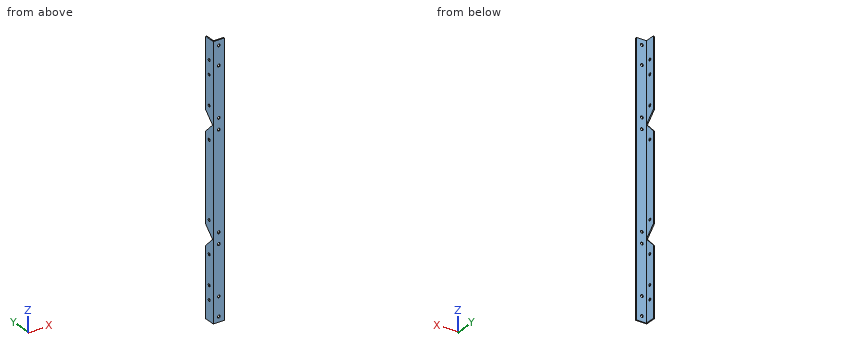
```python
from build123d import *

# Parameters (mm, degrees)
BOSS_EXTRUDE1_DEPTH = 208.28
SKETCH2_R           = 2.38125
CUT_EXTRUDE1_DEPTH  = 1.778
SKETCH3_W           = 1.778
SKETCH3_H           = 17.272
BOSS_EXTRUDE2_DEPTH = 20.32
SKETCH4_R           = 2.38125
CUT_EXTRUDE2_DEPTH  = 1.778


with BuildPart() as part:
    # Sketch1 → Boss-Extrude1 (new body)
    with BuildSketch(Plane.XY):
        Polygon((0, 0), (0, 17.272), (-1.778, 17.272), (-1.778, -1.778), (17.272, -1.778), (17.272, 0), align=None)
    boss_extrude1 = extrude(amount=BOSS_EXTRUDE1_DEPTH)

    # Sketch2 → Cut-Extrude1 (cut)
    with BuildSketch(Plane(origin=(0, 0, 0), x_dir=(0, 0, -1), z_dir=(1, 0, 0))):
        with Locations(Location((-194.31, 8.636, 0), (0, 0, 90))):
            Circle(SKETCH2_R)
        with Locations(Location((-170.434, 8.636, 0), (0, 0, 90))):
            Circle(SKETCH2_R)
        with Locations(Location((-120.269, 8.636, 0), (0, 0, 90))):
            Circle(SKETCH2_R)
        with Locations(Location((-64.897, 8.636, 0), (0, 0, 90))):
            Circle(SKETCH2_R)
        Polygon((-92.583, 0), (-109.855, 17.272), (-75.311, 17.272), align=None)
    cut_extrude1 = extrude(amount=-CUT_EXTRUDE1_DEPTH, mode=Mode.SUBTRACT)

    # Sketch3 → Boss-Extrude2 (add)
    with BuildSketch(Plane.XY.offset(208.28)):
        Polygon((-1.778, 0), (-1.778, -1.778), (17.272, -1.778), (17.272, 0), (0, 0), align=None)
        with Locations((-0.889, 8.636)):
            Rectangle(SKETCH3_W, SKETCH3_H)
    boss_extrude2 = extrude(amount=BOSS_EXTRUDE2_DEPTH)

    # Sketch4 → Cut-Extrude2 (cut)
    with BuildSketch(Plane(origin=(0, 0, 0), x_dir=(1, 0, 0), z_dir=(0, 1, 0))):
        with Locations(Location((7.747, -219.456, 0), (0, 0, 180))):
            Circle(SKETCH4_R)
        with Locations(Location((7.747, -83.058, 0), (0, 0, 180))):
            Circle(SKETCH4_R)
        with Locations(Location((7.747, -102.108, 0), (0, 0, 180))):
            Circle(SKETCH4_R)
        with Locations(Location((7.747, -186.944, 0), (0, 0, 180))):
            Circle(SKETCH4_R)
    cut_extrude2 = extrude(amount=-CUT_EXTRUDE2_DEPTH, mode=Mode.SUBTRACT)

    # Mirror3: Boss-Extrude1, Cut-Extrude1, Boss-Extrude2, Cut-Extrude2 across plane
    add(boss_extrude1.mirror(Plane(origin=(0, 0, 0), x_dir=(1, 0, 0), z_dir=(0, 0, -1))))
    add(cut_extrude1.mirror(Plane(origin=(0, 0, 0), x_dir=(1, 0, 0), z_dir=(0, 0, -1))), mode=Mode.SUBTRACT)
    add(boss_extrude2.mirror(Plane(origin=(0, 0, 0), x_dir=(1, 0, 0), z_dir=(0, 0, -1))))
    add(cut_extrude2.mirror(Plane(origin=(0, 0, 0), x_dir=(1, 0, 0), z_dir=(0, 0, -1))), mode=Mode.SUBTRACT)


solid = part.part
```
For this review, take the finished solid that the model builds, in its own axes (mm). Round coordinates to 2 decimals unless told otherwise and drop trailing zeros. Write each loop counter-clockwise with the first axis right and the second up, starting at its lowest first coordinate (ties: lowest second). Pieces come first, ordered by that corner, then holes. Notation, with made-up numbers: (-7, -3.75) -> (12, -3.75) arc R8 cw to (12, 2.25) -> close; hole circle Ø1 at (21.25, -29). An arc over 180 degrees is marked (long way). One line per question, with ' | ' between items. Start each with the question number.
(1) For line 1 along Y through (x, z) = (13, 167), list the stretches that pass through material, from the lowest coordinate up. Write a range as from..to.
(2) Insertion check: P1, Ø2, axis at y = 5, z = -154.5, coming from the +X side; P2, Ø1.5, axis at x = 5, z = 141.5, coming from the +Y side. Each pin has a flat end and moves straight along its axis. Give the tip position at first contact, or say it passes through.
(3) Add section B-B, the plane x = 13.75. Write out the cut boundary in (y, z).
(4) Add section A-A, the plane z = -134. Write out the cut boundary in (x, y), plus the area to 3 significant figures.
Answer list:
1) line 1: -1.78..0
2) P1: x = 0 | P2: y = 0
3) outline: (-1.78, -228.6) -> (0, -228.6) -> (0, 228.6) -> (-1.78, 228.6) -> close
4) outline: (-1.78, -1.78) -> (17.27, -1.78) -> (17.27, 0) -> (0, 0) -> (0, 17.27) -> (-1.78, 17.27) -> close | area: 64.6 mm²
